```python
from build123d import *

# Parameters (mm, degrees)
BOSS_EXTRUDE1_DEPTH = 1.5875
FILLET1_R           = 1.27
CUT_EXTRUDE1_DEPTH  = 58.360405638
LPATTERN1_COUNT     = 16
LPATTERN1_PITCH     = 4.445
SKETCH4_R           = 7.686089714
CUT_EXTRUDE2_DEPTH  = 58.360405641


with BuildPart() as part:
    # Sketch1 → Boss-Extrude1 (new, symmetric)
    with BuildSketch(Plane.XY):
        with BuildLine():
            Line((-38.1, 0), (38.1, 0))
            Line((38.1, 0), (33.02, 5.08))
            Line((33.02, 5.08), (-38.1, 5.08))
            ThreePointArc((-38.1, 5.08), (-44.280636145, 7.357561705), (-47.505517918, 13.101052632))
            ThreePointArc((-47.505517918, 13.101052632), (-49.552624359, 15.197809), (-52.213360556, 13.97))
            ThreePointArc((-52.213360556, 13.97), (-55.276019825, 2.54), (-52.213360556, -8.89))
            ThreePointArc((-52.213360556, -8.89), (-49.552624359, -10.117809), (-47.505517918, -8.021052632))
            ThreePointArc((-47.505517918, -8.021052632), (-44.280636145, -2.277561705), (-38.1, 0))
        make_face()
    extrude(amount=BOSS_EXTRUDE1_DEPTH, both=True)

    # Fillet1
    fillet1_edges = [part.edges().sort_by_distance(p)[0] for p in [
        (-2.54, 5.08, -1.5875),
        (0, 0, -1.5875),
        (-44.280636145, -2.277561705, -1.5875),
        (-2.54, 5.08, 1.5875),
        (-44.280636145, 7.357561705, 1.5875),
        (-49.552624359, 15.197809, 1.5875),
        (-55.276019825, 2.54, 1.5875),
        (-49.552624359, -10.117809, 1.5875),
        (-44.280636145, -2.277561705, 1.5875),
        (-49.552624359, -10.117809, -1.5875),
        (0, 0, 1.5875),
        (-55.276019825, 2.54, -1.5875),
        (-49.552624359, 15.197809, -1.5875),
        (-44.280636145, 7.357561705, -1.5875),
    ]]
    fillet(fillet1_edges, radius=FILLET1_R)

    # Sketch3 → Cut-Extrude1 (cut, symmetric)
    with BuildSketch(Plane.XY):
        with BuildLine():
            Line((30.592919151, 2.921), (31.637080849, 2.921))
            ThreePointArc((31.637080849, 2.921), (32.190091062, 4.089181925), (33.02, 5.08))
            Line((33.02, 5.08), (29.21, 5.08))
            ThreePointArc((29.21, 5.08), (30.039908938, 4.089181925), (30.592919151, 2.921))
        make_face()
    cut_extrude1 = extrude(amount=CUT_EXTRUDE1_DEPTH, both=True, mode=Mode.SUBTRACT)

    # LPattern1: Cut-Extrude1 ×16
    with Locations(*[(-i * LPATTERN1_PITCH, 0, 0) for i in range(1, LPATTERN1_COUNT)]):
        add(cut_extrude1, mode=Mode.SUBTRACT)

    # Sketch4 → Cut-Extrude2 (cut, through all)
    with BuildSketch(Plane(origin=(0, 0, 0), x_dir=(0, 0, -1), z_dir=(1, 0, 0))):
        Circle(SKETCH4_R)
    extrude(amount=CUT_EXTRUDE2_DEPTH, mode=Mode.SUBTRACT)


solid = part.part
```
Build history of the part. All positions in model axes, mm. A direction names the side the tool comes from. Give positions to 0.01 mm unless a question says otherwise; leave off trailing zeros.
1) Drop flat-ended pins along their axis: P1, Ø0.7, axis at x = -7, z = 0, coming from the +Y side; P2, Ø0.8, axis at x = -4.5, z = -1, coming from the +Y side; P3, Ø1.5, axis at x = -31.5, y = -2.5, coming from the +Z side; P4, Ø1.5, axis at y = 10, z = 1, coming from the +X side. Give the stop position or say it passes through.
Values follow:
P1: stops at y = 5.08
P2: stops at y = 2.92
P3: passes through
P4: stops at x = -46.09
2) 3-axis set-ups, long thin cutter, end or side, ignore diameter. For faces 1 (the face through (-24.47, 4.55, 1.35)), 2 (the face through (-16.7, 4.1, 0)), 3 (the face through (-15.58, 4.55, -1.35)): which of +Z, -Z, +X, -X, +Y, -Y reach the whole face in a straight line?
Values follow:
face 1: +Z, +X, +Y
face 2: +Z, -Z, +Y
face 3: -Z, +X, +Y
3) Probe line 1 along Y through (x, z) = (-22, -0.35); line 2 along Y through (x, z) = (-24.5, 0); line 3 along X through (y, z) = (1.25, 0.1). List the from-to ranges inside material, lowest first.
Values follow:
line 1: y = 0 to 2.92
line 2: y = 0 to 5.08
line 3: x = -55.24 to 0
